Print and shaded views of the part. All mm, measured from the part's lowest x, y and z. Give positions to 0.01 mm unless a question says otherwise; leave off trailing zeros. Loops run counter-clockwise (first coordinate to the right, second up) from the corner with the lowest first, then second, coordinate; pieces in that order, holes last. Notation, with made-up numbers: M 40,-18 L 73,-18 A33 cw 73,18 Z; hole C 79,89.5 d11. An arc over 180 degrees is marked long. Answer in a Markdown table with one row per item.
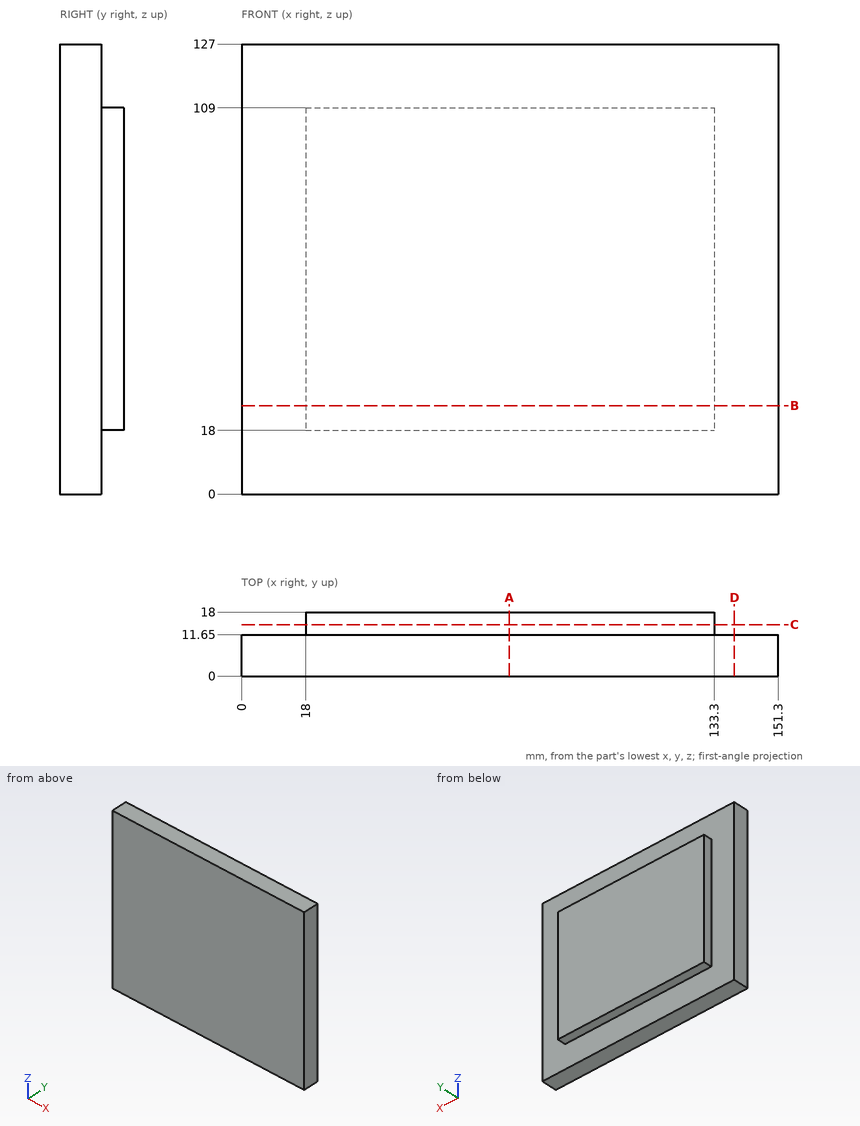
(1) Saw through at B-B, the plane z = 25. Give the cut face in (x, y), and give its area (3 significant figures).
Established:
| item | result |
|---|---|
| outline | M 0,0 L 151.3,0 L 151.3,11.65 L 133.3,11.65 L 133.3,18 L 18,18 L 18,11.65 L 0,11.65 Z |
| area | 2,490 mm2 |
(2) Saw through at A-A, the plane x = 75.5. Give the cut face in (y, z).
Established:
| item | result |
|---|---|
| outline | M 0,0 L 11.65,0 L 11.65,18 L 18,18 L 18,109 L 11.65,109 L 11.65,127 L 0,127 Z |
(3) Flat gauge pins, fed straight in: P1, Ø3, axis at x = 72, y = 13.5, coming from the -Z side; P2, Ø1.9, axis at y = 13.5, z = 42.5, coming from the +X side. Where does each tip first touch, or does it go through?
Established:
| item | result |
|---|---|
| P1 | stops at z = 18 |
| P2 | stops at x = 133.3 |
(4) Saw through at D-D, the plane x = 139. Give the cut face in (y, z), and give its area (3 significant figures).
Established:
| item | result |
|---|---|
| outline | M 0,0 L 11.65,0 L 11.65,127 L 0,127 Z |
| area | 1,480 mm2 |
(5) Wall check: L1, parallel to Z at x = 131.5, y = 12.75; L2, parallel to Y at x = 136, z = 17; L3, parallel to X at y = 15, z = 73. Give the ranges that are in metal, low to high.
Established:
| item | result |
|---|---|
| L1 | z = 18 to 109 |
| L2 | y = 0 to 11.65 |
| L3 | x = 18 to 133.3 |
(6) Saw through at C-C, the plane y = 14.5. Give the cut face in (x, z), and give its area (3 significant figures).
Established:
| item | result |
|---|---|
| outline | M 18,18 L 133.3,18 L 133.3,109 L 18,109 Z |
| area | 10,500 mm2 |
